```python
from build123d import *

# Parameters (mm, degrees)
SKETCH1_W            = 52
SKETCH1_H            = 61.2
BOSS_EXTRUDE1_DEPTH  = 2
M6_CLEARANCE_HOLE1_D = 6.6
SKETCH4_W            = 52
SKETCH4_H            = 61.2
BOSS_EXTRUDE2_DEPTH  = 2


with BuildPart() as part:
    # Sketch1 → Boss-Extrude1 (new body)
    with BuildSketch(Plane.XY):
        Rectangle(SKETCH1_W, SKETCH1_H)
    extrude(amount=BOSS_EXTRUDE1_DEPTH)

    # M6 Clearance Hole1 (through all)
    with Locations(Plane.XY.offset(2)):
        with Locations((20, -26.5), (-20, -26.5), (-20, 26.5), (20, 26.5)):
            Hole(M6_CLEARANCE_HOLE1_D / 2)

    # Sketch4 → Boss-Extrude2 (add)
    with BuildSketch(Plane.XY.offset(2)):
        with BuildLine():
            Line((-26, 33.6), (26, 33.6))
            ThreePointArc((26, 33.6), (28.121320344, 32.721320344), (29, 30.6))
            Line((29, 30.6), (29, -30.6))
            ThreePointArc((29, -30.6), (28.121320344, -32.721320344), (26, -33.6))
            Line((26, -33.6), (-26, -33.6))
            ThreePointArc((-26, -33.6), (-28.121320344, -32.721320344), (-29, -30.6))
            Line((-29, -30.6), (-29, 30.6))
            ThreePointArc((-29, 30.6), (-28.121320344, 32.721320344), (-26, 33.6))
        make_face()
        Rectangle(SKETCH4_W, SKETCH4_H, mode=Mode.SUBTRACT)
    extrude(amount=-BOSS_EXTRUDE2_DEPTH)


solid = part.part
```
Can you work these out from the model? Positions are in its coordinate system, mm. Round coordinates to 2 decimals unless told otherwise and drop trailing zeros. Loops run counter-clockwise (first coordinate to the right, second up) from the corner with the lowest first, then second, coordinate; pieces in that order, holes last.
Item 1: Suppose I cut it at B-B, the plane x = -20. Write out the boundary of the cut face in (y, z).
Item 2: Will this pin go through, and if not, where does the flat tip stop? pin 1 Ø4 at (x, y) = (20, 26.5) entering from -Z.
Item 3: Suppose I cut it at A-A, the plane z = 0.7. Write out the boundary of the cut face in (x, y), then the cut area to 3 significant figures.
Item 4: Suppose I cut it at C-C, the plane y = 26.5. Write out the boundary of the cut face in (x, z).
Item 5: If we mould it in two halves opening along Y, with no side actions, what happens to faces 1 (the flat face through (0, 0, 0)), 2 (the cylindrical face through (16.95, -27.76, 0.99)), 3 (the flat face through (0, 33.6, 1))? For each: +Y half, -Y half, draft (parallel to the pull), parting line (faces both ways), or undercut.
Item 6: Please list where these lines run through material, in increasing order: L1, parallel to Y at x = -20, z = 1.05; L2, parallel to Y at x = -19, z = 1.6.
Reported:
1. outline: (-33.6, 0) - (-29.8, 0) - (-29.8, 2) - (-33.6, 2) - close; (-23.2, 0) - (23.2, 0) - (23.2, 2) - (-23.2, 2) - close; (29.8, 0) - (33.6, 0) - (33.6, 2) - (29.8, 2) - close
2. pin 1: passes through
3. outline: (-29, -30.6) arc R3 ccw to (-26, -33.6) - (26, -33.6) arc R3 ccw to (29, -30.6) - (29, 30.6) arc R3 ccw to (26, 33.6) - (-26, 33.6) arc R3 ccw to (-29, 30.6) - close; hole circle Ø6.6 at (-20, -26.5); hole circle Ø6.6 at (-20, 26.5); hole circle Ø6.6 at (20, -26.5); hole circle Ø6.6 at (20, 26.5)
3. area: 3,750 mm2
4. outline: (-29, 0) - (-23.3, 0) - (-23.3, 2) - (-29, 2) - close; (-16.7, 0) - (16.7, 0) - (16.7, 2) - (-16.7, 2) - close; (23.3, 0) - (29, 0) - (29, 2) - (23.3, 2) - close
5. face 1: draft
5. face 2: undercut
5. face 3: +Y half
6. L1: y = -33.6 to -29.8, -23.2 to 23.2, 29.8 to 33.6
6. L2: y = -33.6 to -29.64, -23.36 to 23.36, 29.64 to 33.6
